Check sheet for the modelled part. Datum: model origin and axes. Units: mm. Coordinates: 2 decimals unless noted, no trailing zeros. Order: outer loops, then holes, each group sorted by start corner. A loop starts at its lowest first (then second) coordinate and runs counter-clockwise, first axis right, second up.
Autodesk Inventor part; units mm, degrees
ref_plane "YZ Plane" through (0, 0, 0) normal (1, 0, 0) x (0, 1, 0)
ref_plane "XZ Plane" through (0, 0, 0) normal (0, 1, 0) x (-1, 0, 0)
ref_plane "XY Plane" through (0, 0, 0) normal (0, 0, 1) x (1, 0, 0)
sketch "Sketch1" plane through (0, 0, 0) normal (0, 0, 1) x (1, 0, 0)
  line L0 (0, 0) -> (63.5, 0)
  line L1 (63.5, 0) -> (63.5, 38.1)
  line L2 (38.1, 63.5) -> (0, 63.5)
  line L3 (-25.4, 38.1) -> (-25.4, 0)
  line L4 (-25.4, 0) -> (0, 0)
  line L5 (38.1, 63.5) -> (63.5, 38.1)
  line L6 (0, 63.5) -> (-25.4, 38.1)
  circle A0 centre (-6.35, 12.7) radius 3.2512
  circle A1 centre (-6.35, 38.1) radius 3.2512
  circle A2 centre (19.05, 38.1) radius 3.2512
  circle A3 centre (19.05, 12.7) radius 3.2512
  circle A4 centre (44.45, 38.1) radius 3.2512
  circle A5 centre (44.45, 12.7) radius 3.2512
  dimension "d5" = 63.5
  dimension "d6" = 25.4
  dimension "d7" = 38.1
  dimension "d8" = 25.4
  dimension "d9" = 25.4
  dimension "d10" = 38.1
  dimension "d11" = 25.4
  dimension "d12" = 25.4
  dimension "d13" = 38.1
  dimension "d14" = 135
  dimension "d15" = 135
  dimension "d16" = 90
  dimension "d17" = 6.5024
  dimension "d18" = 12.7
  dimension "d19" = 19.05
  dimension "d22" = 25.4
  dimension "d29" = 25.4
extrude "Extrusion1" add sketch "Sketch1" along normal blind 6.35
properties part number "3.5x2.5"
(1) Cross-section at A-A (x = -6.35). Enter the section's corners in (y, z), and give its area (3 significant figures).
Filled in:
outline: (0, 0) - (9.45, 0) - (9.45, 6.35) - (0, 6.35) - close; (15.95, 0) - (34.85, 0) - (34.85, 6.35) - (15.95, 6.35) - close; (41.35, 0) - (57.15, 0) - (57.15, 6.35) - (41.35, 6.35) - close
area: 280 mm2
(2) Cross-section at B-B (y = 12.7). Enter the section's corners in (x, z).
Filled in:
outline: (-25.4, 0) - (-9.6, 0) - (-9.6, 6.35) - (-25.4, 6.35) - close; (-3.1, 0) - (15.8, 0) - (15.8, 6.35) - (-3.1, 6.35) - close; (22.3, 0) - (41.2, 0) - (41.2, 6.35) - (22.3, 6.35) - close; (47.7, 0) - (63.5, 0) - (63.5, 6.35) - (47.7, 6.35) - close
(3) Thickness scan on probe 1 along X at (y, z) = (14, 4.5); probe 2 along Y at (x, z) = (19.05, 4); probe 3 along Y at (x, z) = (44.45, 3.75). Record the ranges inside material, lowest first.
Filled in:
probe 1: x = -25.4 to -9.33, -3.37 to 16.07, 22.03 to 41.47, 47.43 to 63.5
probe 2: y = 0 to 9.45, 15.95 to 34.85, 41.35 to 63.5
probe 3: y = 0 to 9.45, 15.95 to 34.85, 41.35 to 57.15
(4) Cross-section at C-C (z = 2.75). Enter the section's corners in (x, y).
Filled in:
outline: (-25.4, 0) - (63.5, 0) - (63.5, 38.1) - (38.1, 63.5) - (0, 63.5) - (-25.4, 38.1) - close; hole circle Ø6.5 at (-6.35, 12.7); hole circle Ø6.5 at (-6.35, 38.1); hole circle Ø6.5 at (19.05, 12.7); hole circle Ø6.5 at (19.05, 38.1); hole circle Ø6.5 at (44.45, 12.7); hole circle Ø6.5 at (44.45, 38.1)
(5) Go/stop test with flat-tipped pins: P1, Ø4, axis at x = 19.05, y = 12.7, coming from the -Z side; P2, Ø3, axis at y = 42, z = 2, coming from the -X side. Record where each tip stops, or that it passes through.
Filled in:
P1: passes through
P2: stops at x = -23
(6) Cross-section at D-D (x = 19.05). Enter the section's corners in (y, z).
Filled in:
outline: (0, 0) - (9.45, 0) - (9.45, 6.35) - (0, 6.35) - close; (15.95, 0) - (34.85, 0) - (34.85, 6.35) - (15.95, 6.35) - close; (41.35, 0) - (63.5, 0) - (63.5, 6.35) - (41.35, 6.35) - close
(7) Release check for a two-part mould opening along X. For faces 1 (the cylindrical face through (-8.746, 10.503, 3.131)), 2 (the flat face through (18, 32, 0)), 3 (the flat face through (-25.4, 19, 3)) record: +X half, -X half, draft (parallel to the pull), parting line (faces both ways), or undercut.
Filled in:
face 1: undercut
face 2: draft
face 3: -X half
